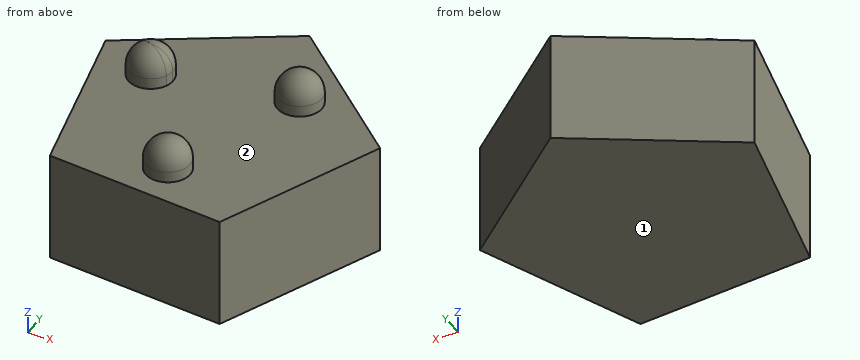
```python
from build123d import *

# Parameters (mm, degrees)
F0_R     = 10
F1_DEPTH = 50
F2_DEPTH = 65
F3_R     = 10


with BuildPart() as f1:
    # F0 (on Top) → F1 (new body)
    with BuildSketch(Plane.XY):
        Polygon((35.9642069631, -59.0012792924), (67.2271022816, 15.9715953944), (5.5844272121, 68.8722681007), (-63.7757364568, 26.5938071741), (-45, -52.4363913769), align=None)
        with Locations((0, -36.73)):
            Circle(F0_R, mode=Mode.SUBTRACT)
        with BuildLine():
            ThreePointArc((-27.689133859, 11.5460757896), (-40.7675370752, 6.1650564331), (-46.1485564317, 19.2434596493))
            ThreePointArc((-46.1485564317, 19.2434596493), (-34.9563356375, 25.2003047486), (-26.9188451453, 15.3947677194))
            ThreePointArc((-26.9188451453, 15.3947677194), (-27.1133081161, 13.4322582116), (-27.689133859, 11.5460757896))
        make_face(mode=Mode.SUBTRACT)
        with Locations((23.9935845951, 27.8100844709)):
            Circle(F0_R, mode=Mode.SUBTRACT)
    extrude(amount=F1_DEPTH)

    # F0 (on Top) → F2 (join)
    with BuildSketch(Plane.XY):
        with BuildLine():
            Line((-27.689133859, 11.5460757896), (-46.1485564317, 19.2434596493))
            ThreePointArc((-46.1485564317, 19.2434596493), (-40.7675370752, 6.1650564331), (-27.689133859, 11.5460757896))
        make_face()
        with BuildLine():
            ThreePointArc((-26.9188451453, 15.3947677194), (-34.9563356375, 25.2003047486), (-46.1485564317, 19.2434596493))
            Line((-46.1485564317, 19.2434596493), (-27.689133859, 11.5460757896))
            ThreePointArc((-27.689133859, 11.5460757896), (-27.1133081161, 13.4322582116), (-26.9188451453, 15.3947677194))
        make_face()
        with Locations((23.9935845951, 27.8100844709)):
            Circle(F0_R)
        with Locations((0, -36.73)):
            Circle(F0_R)
    extrude(amount=F2_DEPTH)

    # F3
    f3_edges = [f1.edges().sort_by_distance(p)[0] for p in [
        (-46.148556, 19.24346, 65),
        (-10, -36.73, 65),
        (13.993585, 27.810084, 65),
    ]]
    fillet(f3_edges, radius=F3_R)


solid = f1.part
```
Geometry check sheet. Reference: the model listing, model coordinates, mm. Face numbers are marked on the shaded views. A direction names the side the tool comes from. Round coordinates to 2 decimals unless told otherwise and drop trailing zeros. Loops run counter-clockwise (first coordinate to the right, second up) from the corner with the lowest first, then second, coordinate; pieces in that order, holes last. Notation, with made-up numbers: M 51,72.5 L 83,72.5 A29 cw 83,110.5 Z; hole C 27,58 d8. An arc over 180 degrees is marked long. Return JSON: item names as keys, results as strings. Group by question number.
(1) Section check C-C, the plane y = 30.5. Enter the section's corners in (x, z) (3 decimals).
(2) Section check A-A, the plane z = 14.5. Enter the section's corners in (x, y).
(3) Section check D-D, the plane z = 61.5. Enter the section's corners in (x, y), and give its area (3 significant figures).
(4) Go/stop test with flat-tipped pins: pin 1 (8 mm diameter, centred on y = -37, z = 35, fed in from +X); pin 2 (12 mm diameter, centred on y = -37.5, z = 56.5, fed in from -X); pin 3 (8 mm diameter, centred on y = 11.5, z = 33.5, fed in from -X). Record where each tip stops, or that it passes through.
(5) Scan lines: line 1 along Z through (x, y) = (8, -43.5); line 2 along X through (y, z) = (19, 51); line 3 along Y through (x, z) = (-18, 28). Record each from-to range of solid material in increasing order. Write a range as [from, to].
(6) Section check B-B, the plane x = 0. Enter the section's corners in (y, z).
(7) Set-up check for the marked faces 1 and 2: record each of +Z, -Z, +X, -X, +Y, -Y from which the full face is reachable in a straight line by a thin tool's end or side.
Data:
{
 "1": {"outline": "M -57.367,0 L 50.298,0 L 50.298,50 L 33.625,50 L 33.625,55 A9.631 ccw 14.362,55 L 14.362,50 L -57.367,50 Z"},
 "2": {"outline": "M -63.78,26.59 L -45,-52.44 L 35.96,-59 L 67.23,15.97 L 5.58,68.87 Z"},
 "3": {"outline": "C -36.92,15.39 d15.2; C 0,-36.73 d15.2; C 23.99,27.81 d15.2", "area": "544 mm²"},
 "4": {"pin 1": "x = 46.81", "pin 2": "x = -10", "pin 3": "x = -61.14"},
 "5": {"line 1": "[0, 50]", "line 2": "[-46.25, -27.59], [19.26, 28.72]", "line 3": "[-54.63, 54.5]"},
 "6": {"outline": "M -56.09,0 L 65.47,0 L 65.47,50 L -26.73,50 L -26.73,55 A10 ccw -46.73,55 L -46.73,50 L -56.09,50 Z"},
 "7": {"face 1": "-Z, +X, -X, +Y, -Y", "face 2": "+Z"}
}
